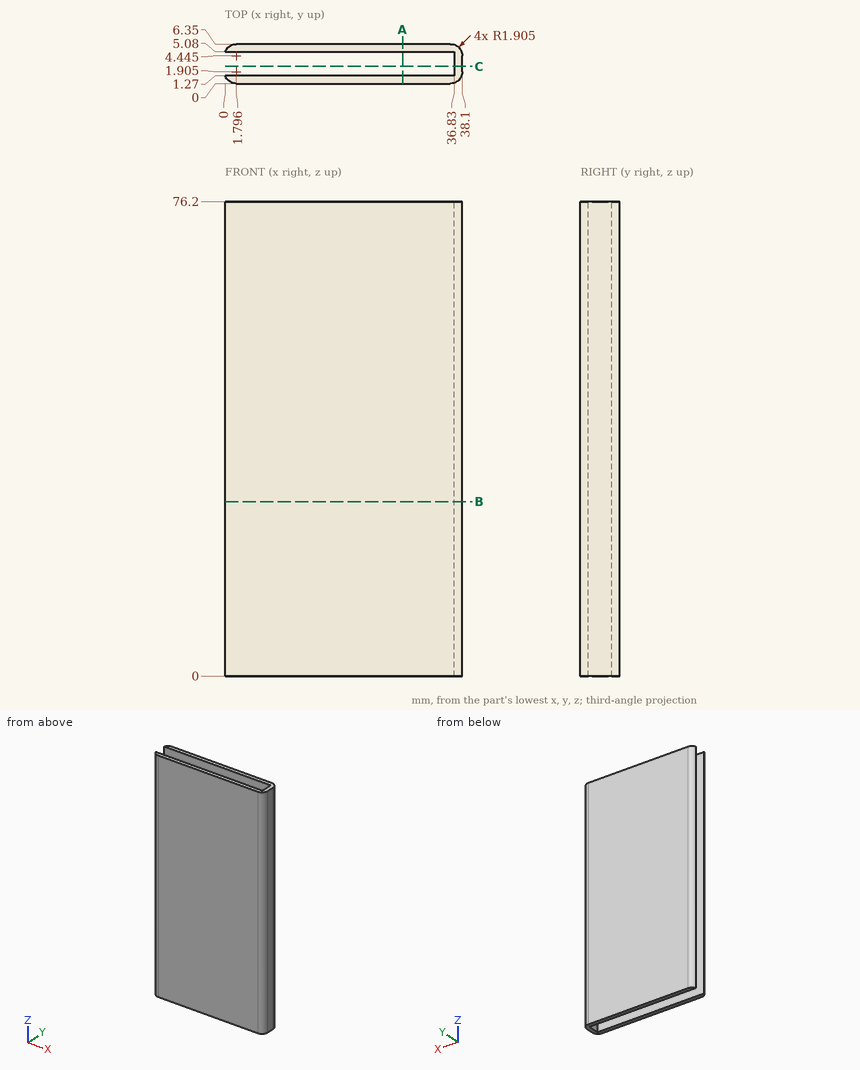
Input: dimensioned drawing with shaded views. Units: mm. Origin: part minimum x, y, z. Round coordinates to 2 decimals unless told otherwise and drop trailing zeros. Order: outer loops, then holes, each group sorted by start corner. A loop starts at its lowest first (then second) coordinate and runs counter-clockwise, first axis right, second up. Notation, with made-up numbers: (-29.75, -17.75) - (2.25, -17.75) arc R5 ccw to (2.25, -8.75) - close; hole circle Ø7 at (-2.75, -14.75). An arc over 180 degrees is marked (long way). Write item = value, one per line. Start each with the question number.
Q1. Pin query (flat end, axial travel): pin 1 (1.9 mm diameter, centred on y = 4, z = 31, fed in from -X). Return the tip coordinate at first contact, or that it passes through.
Q2. Cut plane A-A on x = 28.5. Return the cut outline in (y, z).
Q3. Ray query, line 1 (Y direction, x = 31, z = 32.5); line 2 (X direction, y = 4.5, z = 54); line 3 (X direction, y = 1, z = 18.5). Return the intervals inside material, ascending. Write a range as from..to.
Q4. Cut plane C-C on y = 2.75. Return the cut outline in (x, z).
Q5. Cut plane B-B on z = 28. Return the cut outline in (x, y) (3 decimals), and give its area (3 significant figures).
Outcome:
q1.pin_1 = 36.83
q2.outline = (0, 0) - (1.27, 0) - (1.27, 76.2) - (0, 76.2) - close; (5.08, 0) - (6.35, 0) - (6.35, 76.2) - (5.08, 76.2) - close
q3.line_1 = 0..1.27, 5.08..6.35
q3.line_2 = 36.83..38.1
q3.line_3 = 0.12..37.87
q4.outline = (36.83, 0) - (38.1, 0) - (38.1, 76.2) - (36.83, 76.2) - close
q5.outline = (0, 1.27) arc R1.905 ccw to (1.796, 0) - (36.195, 0) arc R1.905 ccw to (38.1, 1.905) - (38.1, 4.445) arc R1.905 ccw to (36.195, 6.35) - (1.796, 6.35) arc R1.905 ccw to (0, 5.08) - (36.83, 5.08) - (36.83, 1.27) - close
q5.area = 98.8 mm^2
